Source: CAD feature listing. Evaluate the final solid. Frame: model axes, mm. Face numbers are marked on the shaded views. A direction names the side the tool comes from. Round coordinates to 2 decimals unless told otherwise and drop trailing zeros. Order: outer loops, then holes, each group sorted by start corner. A loop starts at its lowest first (then second) coordinate and runs counter-clockwise, first axis right, second up. Notation, with made-up numbers: (56.25, 34) -> (94.25, 34) arc R4 ccw to (94.25, 39) -> close; hole circle Ø6 at (71.25, -39.5). An arc over 180 degrees is marked (long way). One line per item, written item: value. Start each with the question number.
1) Reachability of the marked faces 4, 5 and 6 from +Z, -Z, +X, -X, +Y, -Y: full face, straight path, thin tool, end or side. Return the list, or none.
2) Ray query, L1, parallel to Y at x = 18.5, z = 12.5; L2, parallel to Z at x = 5, y = 49.5; L3, parallel to Y at x = -27.5, z = 5. Return the intervals inside material, ascending.
3) Mould query, pull axis Z, two halves, no side actions, for the marked faces 1, 2 and 3. Classes: pulls with the +Z half, pulls with the -Z half, needs draft (parallel to the pull), parting line crosses it, or undercut.
4) Section B-B (x = -24.5). Return the cut outline in (y, z), and give its area (3 significant figures).
5) Pin query (flat end, axial travel): P1, Ø3, axis at y = 22, z = -9.5, coming from the -X side; P2, Ø6, axis at x = 1.5, z = -9.5, coming from the +Y side; P3, Ø1.8, axis at y = 48.5, z = -6.5, coming from the +X side. Return the tip coordinate at first contact, or that it passes through.
6) Section A-A (y = 29). Return the cut outline in (x, z), and give its area (3 significant figures).
7) Section D-D (x = 23.5). Return the cut outline in (y, z).
8) Section C-C (z = -2). State how many separate pieces and enclosed holes the cut face has, and give its area (3 significant figures).
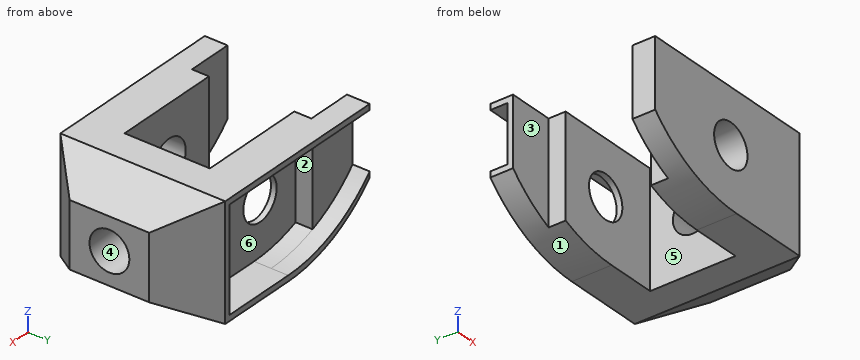
```python
from build123d import *

# Parameters (mm, degrees)
SKETCH1_R           = 7.5
BOSS_EXTRUDE2_DEPTH = 58
CUT_EXTRUDE1_DEPTH  = 29
SKETCH6_R           = 7
CUT_EXTRUDE2_DEPTH  = 64
CUT_EXTRUDE3_DEPTH  = 64
CUT_EXTRUDE7_DEPTH  = 6
CUT_EXTRUDE8_DEPTH  = 6


with BuildPart() as part:
    # Sketch1 → Boss-Extrude2 (new body)
    with BuildSketch(Plane(origin=(0, 0, 0), x_dir=(1, 0, 0), z_dir=(0, 1, 0))):
        with BuildLine():
            Line((0, -19), (31, -19))
            Line((31, -19), (46, -10.339745962))
            Line((46, -10.339745962), (46, 12.339745962))
            Line((46, 12.339745962), (31, 21))
            Line((31, 21), (2.66060556, 21))
            ThreePointArc((2.66060556, 21), (-17.33939444, 16.82575695), (-34, 5))
            Line((-34, 5), (-34, -19))
            Line((-34, -19), (0, -19))
        make_face()
        Circle(SKETCH1_R, mode=Mode.SUBTRACT)
    extrude(amount=BOSS_EXTRUDE2_DEPTH)

    # Sketch4 → Cut-Extrude1 (cut, symmetric)
    with BuildSketch(Plane.XY):
        Polygon((31, 0), (46, 15), (46, 0), align=None)
        Polygon((31, 58), (46, 43), (46, 58), align=None)
    extrude(amount=CUT_EXTRUDE1_DEPTH, both=True, mode=Mode.SUBTRACT)

    # Sketch6 → Cut-Extrude2 (cut, symmetric)
    with BuildSketch(Plane(origin=(0, 0, 0), x_dir=(0, 0, -1), z_dir=(1, 0, 0))):
        with Locations((1, 29)):
            Circle(SKETCH6_R)
    extrude(amount=CUT_EXTRUDE2_DEPTH, both=True, mode=Mode.SUBTRACT)

    # Sketch7 → Cut-Extrude3 (cut, symmetric)
    with BuildSketch(Plane.XY.offset(19)):
        Polygon((-34, 50), (-18, 50), (-18, 44), (20, 44), (20, 14), (-18, 14), (-18, 8), (-34, 8), align=None)
    extrude(amount=CUT_EXTRUDE3_DEPTH, both=True, mode=Mode.SUBTRACT)

    # Sketch8 → Cut-Extrude7 (cut)
    with BuildSketch(Plane(origin=(0, 58, 0), x_dir=(1, 0, 0), z_dir=(0, 1, 0))):
        with BuildLine():
            Line((29, 19), (2.66060556, 19))
            ThreePointArc((2.66060556, 19), (-17.33939444, 14.82575695), (-34, 3))
            Line((-34, 3), (-34, -17))
            Line((-34, -17), (29, -17))
            Line((29, -17), (29, 19))
        make_face()
    extrude(amount=-CUT_EXTRUDE7_DEPTH, mode=Mode.SUBTRACT)

    # Sketch11 → Cut-Extrude8 (cut)
    with BuildSketch(Plane(origin=(0, 52, 0), x_dir=(1, 0, 0), z_dir=(0, 1, 0))):
        with BuildLine():
            Line((-16, -17), (29, -17))
            Line((29, -17), (29, 19))
            Line((29, 19), (2.66060556, 19))
            ThreePointArc((2.66060556, 19), (-6.842943589, 18.088517533), (-16, 15.387302143))
            Line((-16, 15.387302143), (-16, -17))
        make_face()
    extrude(amount=-CUT_EXTRUDE8_DEPTH, mode=Mode.SUBTRACT)


solid = part.part
```
Findings:
1. face 4: +X, -X
1. face 5: +Z, -Z, -X
1. face 6: +Y
2. L1: 0 to 14, 44 to 46
2. L2: -21 to -19, 17 to 19
2. L3: 0 to 8, 50 to 52
3. face 1: pulls with the -Z half
3. face 2: undercut
3. face 3: needs draft
4. outline: (0, -12.98) -> (8, -12.98) -> (8, 19) -> (0, 19) -> close; (50, -12.98) -> (58, -12.98) -> (58, -10.98) -> (52, -10.98) -> (52, 17) -> (58, 17) -> (58, 19) -> (50, 19) -> close
4. area: 344 mm2
5. P1: x = 20
5. P2: y = 46
5. P3: x = 41.4
6. outline: (20, -21) -> (31, -21) -> (46, -12.34) -> (46, -8) -> (20, -8) -> close; (20, 6) -> (46, 6) -> (46, 10.34) -> (31, 19) -> (20, 19) -> close
6. area: 546 mm2
7. outline: (0, -21) -> (58, -21) -> (58, -19) -> (46, -19) -> (46, 17) -> (58, 17) -> (58, 19) -> (0, 19) -> close; hole circle Ø14 at (29, -1)
8. separate pieces: 4
8. enclosed holes: 0
8. area: 1,360 mm2
